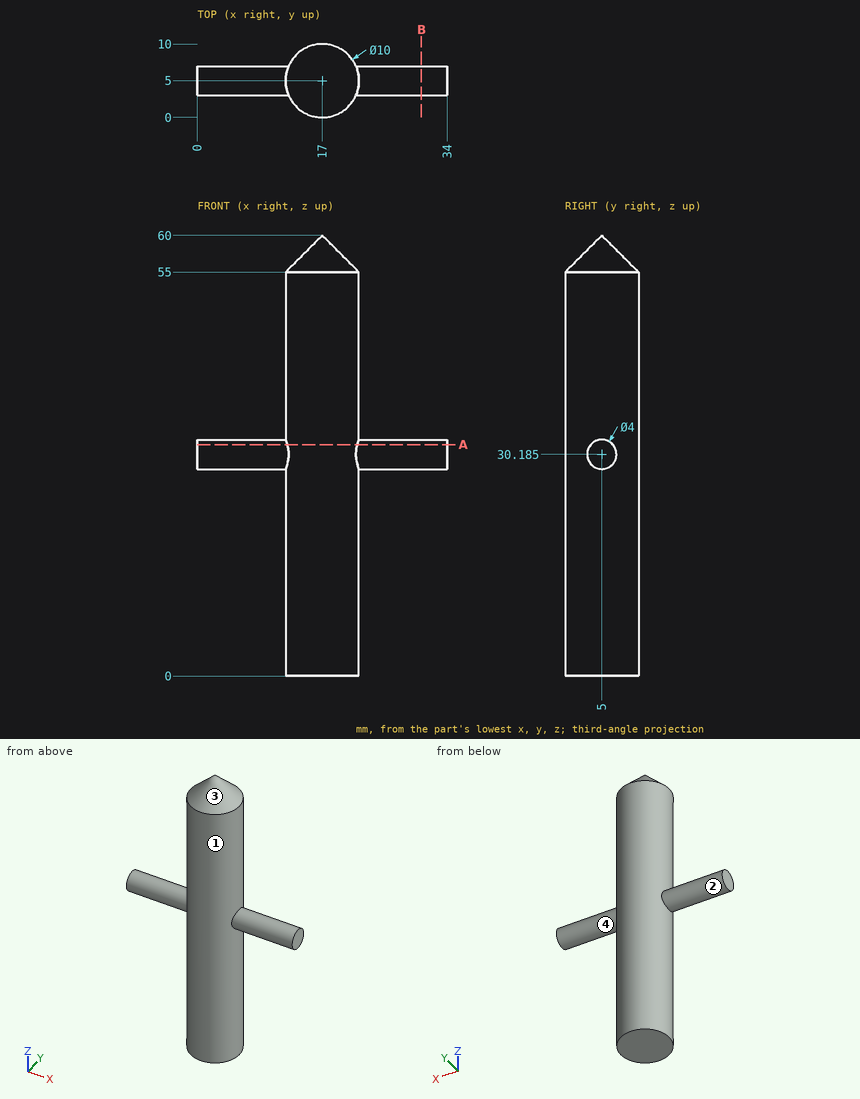
The drawing under review shows one solid part. Ordinate dimensions are in mm from its lowest x, y, z. A direction names the side the tool comes from. Round coordinates to 2 decimals unless told otherwise and drop trailing zeros. Order: outer loops, then holes, each group sorted by start corner. A loop starts at its lowest first (then second) coordinate and runs counter-clockwise, first axis right, second up. Notation, with made-up numbers: (20.5, -35) -> (34.5, -35) arc R29 cw to (34.5, -8) -> close; hole circle Ø3 at (-29.5, 43.5). An arc over 180 degrees is marked (long way). Use a Markdown table: item, result.
Item 1: For pin 1 (1.5 mm diameter, centred on y = 6.5, z = 43, fed in from -X); pin 2 (2 mm diameter, centred on y = 8, z = 31.5, fed in from -X); pin 3 (3 mm diameter, centred on y = 8, z = 17.5, fed in from +X), all flat-tipped, find the tip position at first contact; note any pin that passes through.
Resolved:
| item | result |
|---|---|
| pin 1 | stops at x = 12.06 |
| pin 2 | stops at x = 12.42 |
| pin 3 | stops at x = 21.77 |
Item 2: For line 1 along X through (y, z) = (4.75, 39); line 2 along X through (y, z) = (3, 49.5); line 3 along Y through (x, z) = (13, 52), list the stretches that pass through material, from the lowest coordinate up. Write a range as [from, to].
Resolved:
| item | result |
|---|---|
| line 1 | x = [12.01, 21.99] |
| line 2 | x = [12.42, 21.58] |
| line 3 | y = [2, 8] |
Item 3: Machinability: for the marked faces 3 and 4, which of the approach directions +Z, -Z, +X, -X, +Y, -Y give a long, thin tool a straight path to every point of the face, cutting with its end or side? Answer none if there is none.
Resolved:
| item | result |
|---|---|
| face 3 | +Z |
| face 4 | +X |
Item 4: Take a section at A-A (z = 31.5). State the section outline as (x, y) points, plus the area to 3 significant figures.
Resolved:
| item | result |
|---|---|
| outline | (0, 3.49) -> (12.23, 3.49) arc R5 ccw to (21.77, 3.49) -> (34, 3.49) -> (34, 6.51) -> (21.77, 6.51) arc R5 ccw to (12.23, 6.51) -> (0, 6.51) -> close |
| area | 151 mm² |
Item 5: Draft analysis for pull direction X (two halves, no side actions). For the marked faces 1 and 2, state which applies: +X half, -X half, draft (parallel to the pull), parting line (faces both ways), or undercut.
Resolved:
| item | result |
|---|---|
| face 1 | parting line |
| face 2 | draft |
Item 6: Take a section at B-B (x = 30.5). State the section outline as (y, z) points (1 decimal), plus the area to 3 significant figures.
Resolved:
| item | result |
|---|---|
| outline | circle Ø4 at (5, 30.2) |
| area | 12.6 mm² |
